Autodesk Inventor part; units mm, degrees
ref_plane "YZ Plane" through (0, 0, 0) normal (1, 0, 0) x (0, 1, 0)
ref_plane "XZ Plane" through (0, 0, 0) normal (0, 1, 0) x (-1, 0, 0)
ref_plane "XY Plane" through (0, 0, 0) normal (0, 0, 1) x (1, 0, 0)
sketch "草圖3" plane through (0, 0, 0) normal (0, 1, 0) x (-1, 0, 0)
  line L0 (0, 0) -> (0, -300)
  dimension "d15" = 300
sketch "草圖1" plane through (0, 0, 0) normal (0, 0, 1) x (1, 0, 0)
  line L0 (0, 0) -> (-9.6483, 0) construction
  line L1 (0, 0) -> (0, 9.3404) construction
  line L2 (-8.1216, 4.6307) -> (-8.4962, 8.9128)
  arc A0 (-6.8323, 9.7444) -> (-8.4962, 8.9128) centre (-7.5, 9) ccw
  line L3 (-6.8323, 9.7444) -> (-0.8307, 4.361)
  arc A1 (-4.5, 1) -> (-0.8307, 4.361) centre (-2.5, 2.5) ccw
  line L4 (-4.5, 1) -> (-6, 1)
  line L5 (-6, 1) -> (-8, 0)
  line L6 (-8, 0) -> (-15.9689, 0)
  line L7 (-15.9689, 0) -> (-18.1528, 1)
  line L8 (-18.1528, 1) -> (-101.5326, 1)
  line L9 (-9.6159, 3) -> (-17.1685, 3)
  arc A2 (-9.6159, 3) -> (-8.1216, 4.6307) centre (-9.6159, 4.5) ccw
  line L10 (-19.1004, 4.4824) -> (-19.5385, 6.1176)
  line L11 (-21.4704, 7.5999) -> (-22.2327, 7.5999)
  arc A3 (-19.5385, 6.1176) -> (-21.4704, 7.5999) centre (-21.4704, 5.5999) ccw
  arc A4 (-19.1004, 4.4824) -> (-17.1685, 3) centre (-17.1685, 5) ccw
  line L12 (-14, 16.4786) -> (-11, 16.4786) construction
  line L13 (-11, 16.4786) -> (-11, 4.7787) construction
  line L14 (-11, 4.7787) -> (-14, 4.7787) construction
  line L15 (-14, 4.7787) -> (-14, 16.4786) construction
  arc A5 (-24.139, 8.995) -> (-69.7556, 77.7407) centre (-167.1146, -36.3699) ccw
  arc A6 (-24.139, 8.995) -> (-22.2327, 7.5999) centre (-22.2327, 9.5999) ccw
  line L16 (-69.7556, 77.7407) -> (-101.5326, 77.7407)
  line L17 (-101.5326, 77.7407) -> (-101.5326, 1)
  point P0 (-23.7038, 7.5999)
  point P1 (-12.5, 4.7787)
  dimension "d0" = 10
  dimension "d4" = 1
  dimension "d5" = 2.5
  dimension "d8" = 1.5
  dimension "d9" = 2
  dimension "d10" = 2
  dimension "d11" = 105
  dimension "d13" = 3
  dimension "d14" = 10
  dimension "d20" = 5
  dimension "d21" = 85
  dimension "d22" = 3
  dimension "d24" = 150
  dimension "d25" = 2
  dimension "d26" = 2
  dimension "d27" = 7.9689
  dimension "d28" = 2
  dimension "d29" = 1.5
sweep "掃掠1" add profiles "草圖1" path "草圖3"
fillet "圓角1" radius 2 3 edges at (-6, 1, -150) (-4.5, 1, -150) (-8, 0, -150)
properties part number "0 零件"
Read the model definition and answer for the solid it produces. Units are mm, in the model's axes. A direction names the side the tool comes from. Give positions to 0.01 mm unless a question says otherwise; leave off trailing zeros. Write each loop counter-clockwise with the first axis right and the second up, starting at its lowest first coordinate (ties: lowest second). Pieces come first, ordered by that corner, then holes. Notation, with made-up numbers: (24.5, 60.25) - (71.5, 60.25) arc R37 ccw to (71.5, 96.25) - close; hole circle Ø9 at (56, 54.5). An arc over 180 degrees is marked (long way). Write item = value, one per line. Start each with the question number.
Item 1: A tool of negligible diameter and unlimited length cuts with its end or side. For faces 1 (the flat face through (-12, 0, -152)), 2 (the flat face through (-13, 3, -152)), 3 (the flat face through (-60, 1, -152)), from which of +Z, -Z, +X, -X, +Y, -Y can it reach the whole face along a straight path? Write none if from no direction.
Item 2: Find section B-B (x = -13). Give the vertices of the cut face in (y, z), then the cut area to 3 significant figures.
Item 3: Each of these flat-tipped pins is pushed along its axis until it touches: P1, Ø2, axis at x = -62.5, z = -53, coming from the -Y side; P2, Ø0.6, axis at x = -22, z = -153, coming from the +Y side; P3, Ø2.5, axis at x = -13.5, z = -88.5, coming from the +Y side. Where does it stop, or does it pass through?
Item 4: Find section C-C (y = 50.5). Give the vertices of the cut face in (x, z), then the cut area to 3 significant figures.
Item 5: Find the intervals of material crossed by probe 1 along Y at (x, z) = (-14.5, -120); probe 2 along Y at (x, z) = (-80.5, -55); probe 3 along X at (y, z) = (8, -17), in increasing order. Write a range as [from, to].
Response:
q1.face_1 = +Z, -Z, +X, -X, -Y
q1.face_2 = +Z, -Z, +Y
q1.face_3 = +Z, -Z, -X, -Y
q2.outline = (0, -300) - (3, -300) - (3, 0) - (0, 0) - close
q2.area = 900 mm²
q3.P1 = 1
q3.P2 = 7.6
q3.P3 = 3
q4.outline = (-101.53, -300) - (-44.83, -300) - (-44.83, 0) - (-101.53, 0) - close
q4.area = 17,000 mm²
q5.probe_1 = [0, 3]
q5.probe_2 = [1, 77.74]
q5.probe_3 = [-101.53, -23.43], [-8.42, -4.89]
